Verification items for the finished model (mm, model axes). A direction names the side the tool comes from. Give positions to 0.01 mm unless a question says otherwise; leave off trailing zeros. Loops run counter-clockwise (first coordinate to the right, second up) from the corner with the lowest first, then second, coordinate; pieces in that order, holes last. Notation, with made-up numbers: M -29,59.5 L -18,59.5 A16 ccw -18,86.5 Z; hole C 77,78.5 d11. An arc over 180 degrees is marked long. Put each result on its own line as item: value. Start each with the question number.
from build123d import *

# Parameters (mm, degrees)
SKETCH1_W                = 50
SKETCH1_H                = 15
BOSS_EXTRUDE1_DEPTH      = 2.5
BOSS_EXTRUDE1_DEPTH_BACK = 2.5
SKETCH2_W                = 5
SKETCH2_H                = 15
BOSS_EXTRUDE2_DEPTH      = 30
SKETCH3_W                = 5
SKETCH3_H                = 15
BOSS_EXTRUDE3_DEPTH      = 30
SKETCH4_R                = 1.5
CUT_EXTRUDE1_DEPTH       = 5
SKETCH5_R                = 1.5
CUT_EXTRUDE2_DEPTH       = 5
SKETCH6_R                = 1.5
CUT_EXTRUDE3_DEPTH       = 5
SKETCH7_R                = 1.5
CUT_EXTRUDE5_DEPTH       = 5
SKETCH11_R               = 1.5
CUT_EXTRUDE6_DEPTH       = 5
SKETCH12_R               = 1.5
CUT_EXTRUDE7_DEPTH       = 5


with BuildPart() as part:
    # Sketch1 → Boss-Extrude1 (new body, two sides)
    with BuildSketch(Plane.XY) as boss_extrude1_sk:
        with Locations((-24.404028235, -7.321208471)):
            Rectangle(SKETCH1_W, SKETCH1_H)
    extrude(amount=BOSS_EXTRUDE1_DEPTH)
    extrude(boss_extrude1_sk.sketch, amount=-BOSS_EXTRUDE1_DEPTH_BACK)

    # Sketch2 → Boss-Extrude2 (add)
    with BuildSketch(Plane.XY.offset(2.5)):
        with Locations((-46.904028235, -7.321208471)):
            Rectangle(SKETCH2_W, SKETCH2_H)
    extrude(amount=BOSS_EXTRUDE2_DEPTH)

    # Sketch3 → Boss-Extrude3 (add)
    with BuildSketch(Plane.XY.offset(2.5)):
        with Locations((-1.904028235, -7.321208471)):
            Rectangle(SKETCH3_W, SKETCH3_H)
    extrude(amount=BOSS_EXTRUDE3_DEPTH)

    # Sketch4 → Cut-Extrude1 (cut)
    with BuildSketch(Plane.ZY.offset(49.404028235)):
        with Locations((25, -7.321208471)):
            Circle(SKETCH4_R)
    extrude(amount=-CUT_EXTRUDE1_DEPTH, mode=Mode.SUBTRACT)

    # Sketch5 → Cut-Extrude2 (cut)
    with BuildSketch(Plane.ZY.offset(49.404028235)):
        with Locations((10, -7.321208471)):
            Circle(SKETCH5_R)
    extrude(amount=-CUT_EXTRUDE2_DEPTH, mode=Mode.SUBTRACT)

    # Sketch6 → Cut-Extrude3 (cut)
    with BuildSketch(Plane(origin=(0.595971765, 0, 0), x_dir=(0, 0, -1), z_dir=(1, 0, 0))):
        with Locations((-25, -7.321208471)):
            Circle(SKETCH6_R)
    extrude(amount=-CUT_EXTRUDE3_DEPTH, mode=Mode.SUBTRACT)

    # Sketch7 → Cut-Extrude5 (cut)
    with BuildSketch(Plane(origin=(0.595971765, 0, 0), x_dir=(0, 0, -1), z_dir=(1, 0, 0))):
        with Locations((-10, -7.321208471)):
            Circle(SKETCH7_R)
    extrude(amount=-CUT_EXTRUDE5_DEPTH, mode=Mode.SUBTRACT)

    # Sketch11 → Cut-Extrude6 (cut)
    with BuildSketch(Plane(origin=(0, 0, -2.5), x_dir=(-1, 0, 0), z_dir=(0, 0, -1))):
        with Locations((41.404028235, -3.571208471)):
            Circle(SKETCH11_R)
        with Locations((41.404028235, -11.071208471)):
            Circle(SKETCH11_R)
    extrude(amount=-CUT_EXTRUDE6_DEPTH, mode=Mode.SUBTRACT)

    # Sketch12 → Cut-Extrude7 (cut)
    with BuildSketch(Plane(origin=(0, 0, -2.5), x_dir=(-1, 0, 0), z_dir=(0, 0, -1))):
        with Locations((6.404028235, -7.321208471)):
            Circle(SKETCH12_R)
    extrude(amount=-CUT_EXTRUDE7_DEPTH, mode=Mode.SUBTRACT)


solid = part.part
Q1. Scan lines: L1, parallel to X at y = -8.5, z = 6; L2, parallel to Y at x = 0, z = 10; L3, parallel to Z at x = -7.5, y = -6. Record each from-to range of solid material in increasing order.
Q2. Cross-section at A-A, the plane z = 10. Record the boundary of the cut face in (x, y).
Q3. Cross-section at D-D, the plane x = -29.5. Record the boundary of the cut face in (y, z).
Q4. Cross-section at C-C, the plane y = -13.5. Record the boundary of the cut face in (x, z).
Q5. Release check for a two-part mould opening along X. For faces 1 (the face through (-49.404, -7, 15)), 2 (the face through (-46.9, -7.3, 23.5)), 3 (the face through (-44.404, -7, 17)) record: pulls with the +X half, pulls with the -X half, needs draft (parallel to the pull), parting line crosses it, or undercut.
Q6. Go/stop test with flat-tipped pins: pin 1 (4 mm diameter, centred on x = -40.5, y = -4.5, fed in from +Z); pin 2 (1.8 mm diameter, centred on y = -7.32, z = 10, fed in from +X); pin 3 (3.5 mm diameter, centred on x = -41.4, y = -3.57, fed in from -Z). Record where each tip stops, or that it passes through.
Q7. Cross-section at B-B, the plane z = 17. Record the boundary of the cut face in (x, y), then the cut area to 3 significant figures.
Q8. Set-up check for faces 4 (the face through (-7.21, -6.056, -0.035)), 5 (the face through (-25, -7, 2.5)): record each of +Z, -Z, +X, -X, +Y, -Y from which the full face is reachable in a straight line by a thin tool's end or side.
Ans:
1. L1: x = -49.4 to -44.4, -4.4 to 0.6
1. L2: y = -14.82 to -8.82, -5.82 to 0.18
1. L3: z = -2.5 to 2.5
2. outline: M -49.4,-14.82 L -44.4,-14.82 L -44.4,-8.82 L -49.4,-8.82 Z; M -49.4,-5.82 L -44.4,-5.82 L -44.4,0.18 L -49.4,0.18 Z; M -4.4,-14.82 L 0.6,-14.82 L 0.6,-8.82 L -4.4,-8.82 Z; M -4.4,-5.82 L 0.6,-5.82 L 0.6,0.18 L -4.4,0.18 Z
3. outline: M -14.82,-2.5 L 0.18,-2.5 L 0.18,2.5 L -14.82,2.5 Z
4. outline: M -49.4,-2.5 L 0.6,-2.5 L 0.6,32.5 L -4.4,32.5 L -4.4,2.5 L -44.4,2.5 L -44.4,32.5 L -49.4,32.5 Z
5. face 1: pulls with the -X half
5. face 2: needs draft
5. face 3: undercut
6. pin 1: stops at z = 2.5
6. pin 2: passes through
6. pin 3: stops at z = -2.5
7. outline: M -49.4,-14.82 L -44.4,-14.82 L -44.4,0.18 L -49.4,0.18 Z; M -4.4,-14.82 L 0.6,-14.82 L 0.6,0.18 L -4.4,0.18 Z
7. area: 150 mm^2
8. face 4: +Z, -Z
8. face 5: +Z, +Y, -Y
